```python
from build123d import *

# Parameters (mm, degrees)
F0_W     = 65.433032
F0_H     = 107.144848
F1_DEPTH = 17.78
F2_W     = 65.433032
F2_H     = 45.072302
F3_DEPTH = 17.78
F5_DEPTH = 17.78
F7_DEPTH = 25.4


with BuildPart() as f1:
    # F0 (on Front) → F1 (new body)
    with BuildSketch(Plane.XZ):
        Rectangle(F0_W, F0_H)
    extrude(amount=F1_DEPTH)

    # F2 (on face) → F3 (join)
    with BuildSketch(Plane(origin=(0, 0, -53.572424), x_dir=(1, 0, 0), z_dir=(0, 0, -1))):
        with Locations((0, 22.536151)):
            Rectangle(F2_W, F2_H)
        with BuildLine():
            ThreePointArc((32.716516, 45.072302), (0, 62.674601), (-32.716516, 45.072302))
            Line((-32.716516, 45.072302), (32.716516, 45.072302))
        make_face()
    extrude(amount=F3_DEPTH)

    # F4 (on face) → F5 (cut)
    with BuildSketch(Plane.YZ.offset(32.716516)):
        Polygon((0, -71.352424), (0, -36.141511), (-17.78, -36.141511), (-17.78, -53.572424), (-31.426151, -53.572424), (-31.426151, -71.352424), align=None)
    extrude(amount=-F5_DEPTH, mode=Mode.SUBTRACT)

    # F6 (on face) → F7 (cut)
    with BuildSketch(Plane.XZ.offset(17.78)):
        with BuildLine():
            Line((13.273248, 13.279006), (13.273248, 93.865842))
            Line((13.273248, 93.865842), (-13.273248, 93.865842))
            Line((-13.273248, 93.865842), (-13.273248, 13.279006))
            ThreePointArc((-13.273248, 13.279006), (0, 0.005758), (13.273248, 13.279006))
        make_face()
    extrude(amount=-F7_DEPTH, mode=Mode.SUBTRACT)


solid = f1.part
```
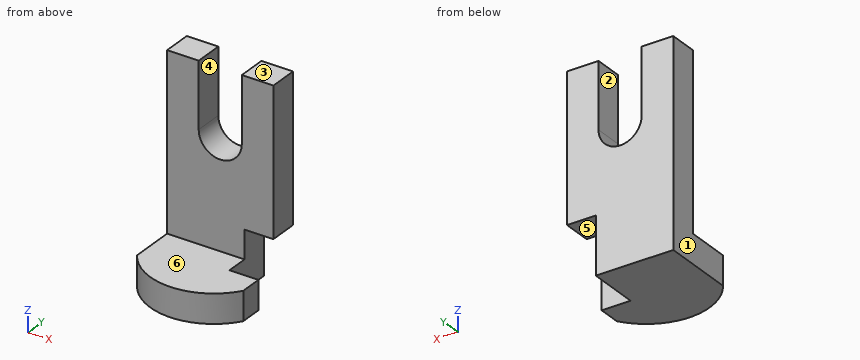
For this review, take the finished solid that the model builds, in its own axes (mm). Face numbers are marked on the shaded views. A direction names the side the tool comes from. Give positions to 0.01 mm unless a question says otherwise; leave off trailing zeros. Loops run counter-clockwise (first coordinate to the right, second up) from the corner with the lowest first, then second, coordinate; pieces in that order, holes last. Notation, with made-up numbers: M 25.25,-0.75 L 56.25,-0.75 A8 cw 56.25,12.25 Z; hole C 46,-8.5 d4. An arc over 180 degrees is marked long. One line per item, written item: value. Start each with the question number.
Q1. Machinability: for the marked faces 4, 5 and 6, which of the approach directions +Z, -Z, +X, -X, +Y, -Y give a long, thin tool a straight path to every point of the face, cutting with its end or side? Answer none if there is none.
Q2. Add section D-D (z = -47.5). Give the boundary of the cut face in (x, y).
Q3. Clearance check with flat-ended pins moving along their axes: pin 1 Ø9 at (x, y) = (20, -9) entering from -Z; pin 2 Ø9 at (x, z) = (26.5, -65.5) entering from +Y; pin 3 Ø8 at (x, y) = (7, -37.5) entering from +Z. State where each tip first meets the part, or that it passes through.
Q4. Add section A-A (z = 36.5). Give the boundary of the cut face in (x, y), and give its area (3 significant figures).
Q5. Add section B-B (x = 27). Give the boundary of the cut face in (y, z).
Q6. Draft analysis for pull direction X (two halves, no side actions). For the marked faces 1, 2 and 3, state which applies: released by +X, released by -X, zero draft, split by the parting line, or undercut.
Q7. For L1, parallel to Y at x = 23.5, z = 40; L2, parallel to Z at x = -9.5, y = -19; L3, parallel to X at y = -10.5, z = 37, list the stretches that pass through material, from the lowest coordinate up.
Q8. Add section C-C (x = 0). Give the boundary of the cut face in (y, z), and give its area (3 significant figures).
Reply:
1. face 4: +Z, +Y, -Y
1. face 5: -Z, +X, +Y, -Y
1. face 6: +Z, +X, -X, -Y
2. outline: M -32.72,-17.78 L 14.94,-17.78 L 14.94,0 L -32.72,0 Z
3. pin 1: z = -36.14
3. pin 2: y = -31.43
3. pin 3: z = -53.57
4. outline: M -32.72,-17.78 L -13.27,-17.78 L -13.27,0 L -32.72,0 Z; M 13.27,-17.78 L 32.72,-17.78 L 32.72,0 L 13.27,0 Z
4. area: 691 mm²
5. outline: M -51.9,-71.35 L -31.43,-71.35 L -31.43,-53.57 L -51.9,-53.57 Z; M -17.78,-36.14 L 0,-36.14 L 0,53.57 L -17.78,53.57 Z
6. face 1: released by -X
6. face 2: undercut
6. face 3: zero draft
7. L1: -17.78 to 0
7. L2: -71.35 to -53.57
7. L3: -32.72 to -13.27, 13.27 to 32.72
8. outline: M -62.67,-71.35 L 0,-71.35 L 0,0.01 L -17.78,0.01 L -17.78,-53.57 L -62.67,-53.57 Z
8. area: 2,070 mm²
